Geometry check sheet. Reference: the model listing, model coordinates, mm. Face numbers are marked on the shaded views. A direction names the side the tool comes from. Round coordinates to 2 decimals unless told otherwise and drop trailing zeros. Order: outer loops, then holes, each group sorted by start corner. A loop starts at its lowest first (then second) coordinate and runs counter-clockwise, first axis right, second up. Notation, with made-up numbers: (46.25, -24) - (59.25, -24) arc R26 ccw to (59.25, 5) - close; hole circle Ø10 at (32, 58.5). An arc over 180 degrees is marked (long way). Return JSON: item names as keys, results as strings. Group by question number.
Q1. Sectioned sample at A-A, the plane y = 15.75. Record the cut outline in (x, z).
Q2. Material ranges on line 1 along Z through (x, y) = (7.5, 1.1); line 2 along X through (y, z) = (7.75, -28); line 3 along X through (y, z) = (21, -21), recorded low to high.
Q3. Tool access check on the marked faces 5 and 6. Record the directions out of +Z, -Z, +X, -X, +Y, -Y that give a thin tool (end or side, any length) a straight path to the whole face; none if there is none.
Q4. Sectioned sample at C-C, the plane x = 21.5. Record the cut outline in (y, z).
Q5. Gauge pin test, flat ends, axial feed: pin 1 Ø3 at (x, y) = (45, 14) entering from +Z (3 decimals); pin 2 Ø2.5 at (y, z) = (7.5, -5) entering from +X; pin 3 Ø8 at (x, z) = (43, -34) entering from +Y; pin 4 Ø3 at (x, z) = (64.5, -5.78) entering from +Y. Record the tip position at first contact, or that the pin passes through.
Q6. Sectioned sample at D-D, the plane z = -6. Record the cut outline in (x, y), then the cut area to 3 significant figures.
Q7. Sectioned sample at B-B, the plane z = -21. Record the cut outline in (x, y), then the cut area to 3 significant figures.
Q8. Draft check along X on the marked faces 1, 2, 3 and 4. Enter one of: pulls with the +X half, pulls with the -X half, needs draft (parallel to the pull), parting line crosses it, or undercut.
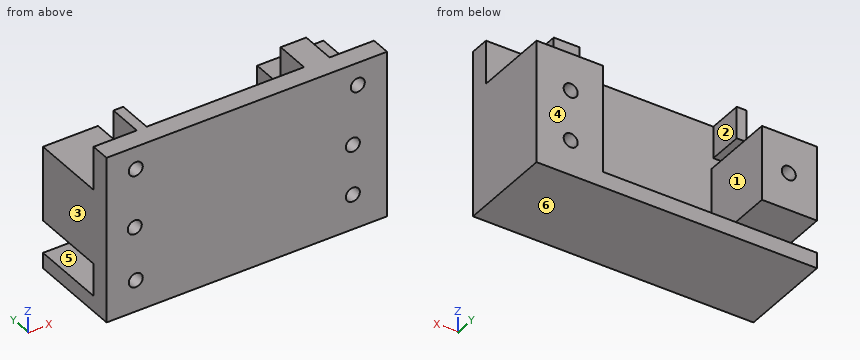
```python
from build123d import *

# Parameters (mm, degrees)
SKETCH2_W                = 72
SKETCH2_H                = 40
BOSS_EXTRUDE1_DEPTH      = 5
BOSS_EXTRUDE2_DEPTH      = 19.5
BOSS_EXTRUDE2_DEPTH_BACK = 5
SKETCH3_W                = 14.135898402
SKETCH3_H                = 19.186853455
CUT_EXTRUDE1_START       = 19.5
SKETCH4_R                = 1.8
CUT_EXTRUDE1_DEPTH       = 30
SKETCH8_W                = 2.527236714
SKETCH8_H                = 8.177193873
SKETCH8_W_2              = 6.563624393
BOSS_EXTRUDE7_DEPTH      = 9
SKETCH9_R                = 1.8
CUT_EXTRUDE2_DEPTH       = 53


with BuildPart() as part:
    # Sketch2 → Boss-Extrude1 (new body)
    with BuildSketch(Plane(origin=(0, 0, 0), x_dir=(1, 0, 0), z_dir=(0, 1, 0))):
        with Locations((36, 20)):
            Rectangle(SKETCH2_W, SKETCH2_H)
    extrude(amount=BOSS_EXTRUDE1_DEPTH)

    # Sketch3 → Boss-Extrude2 (add, two sides: drawn at the far end of the back side and taken through both)
    with BuildSketch(Plane(origin=(0, 5, 0), x_dir=(1, 0, 0), z_dir=(0, 1, 0)).offset(-BOSS_EXTRUDE2_DEPTH_BACK)):
        with Locations((7.067949201, 20.793426728)):
            Rectangle(SKETCH3_W, SKETCH3_H)
        Polygon((55, 38.754979203), (55, 11.2), (72, 11.2), (72, 42.754979203), (0, 42.754979203), (0, 38.754979203), align=None)
    extrude(amount=BOSS_EXTRUDE2_DEPTH + BOSS_EXTRUDE2_DEPTH_BACK)

    # Sketch4 → Cut-Extrude1 (cut)
    with BuildSketch(Plane(origin=(0, 5, 0), x_dir=(1, 0, 0), z_dir=(0, 1, 0)).offset(CUT_EXTRUDE1_START)):
        with Locations(Location((7.5, 34.648486257, 0), (0, 0, 90))):
            Circle(SKETCH4_R)
        with Locations(Location((7.5, 5.778304463, 0), (0, 0, 90))):
            Circle(SKETCH4_R)
        with Locations(Location((64.5, 5.778304463, 0), (0, 0, 90))):
            Circle(SKETCH4_R)
    extrude(amount=-CUT_EXTRUDE1_DEPTH, mode=Mode.SUBTRACT)

    # Sketch8 → Boss-Extrude7 (add)
    with BuildSketch(Plane(origin=(0, 5, 0), x_dir=(1, 0, 0), z_dir=(0, 1, 0))):
        with Locations((12.356862163, 4.088596937)):
            Rectangle(SKETCH8_W, SKETCH8_H)
        with Locations((57.312199978, 4.088596937)):
            Rectangle(SKETCH8_W_2, SKETCH8_H)
    extrude(amount=BOSS_EXTRUDE7_DEPTH)

    # Sketch9 → Cut-Extrude2 (cut)
    with BuildSketch(Plane(origin=(0, 24.5, 0), x_dir=(1, 0, 0), z_dir=(0, 1, 0))):
        with Locations(Location((7.244076977, 20.809705714, 0), (0, 0, 270))):
            Circle(SKETCH9_R)
        with Locations(Location((63.234445615, 20.809705714, 0), (0, 0, 270))):
            Circle(SKETCH9_R)
        with Locations(Location((63.234445615, 33.7549792, 0), (0, 0, 270))):
            Circle(SKETCH9_R)
    extrude(amount=-CUT_EXTRUDE2_DEPTH, mode=Mode.SUBTRACT)


solid = part.part
```
Reply:
{
 "1": {"outline": "(0, -42.75) - (72, -42.75) - (72, -11.2) - (55, -11.2) - (55, -38.75) - (0, -38.75) - close; (0, -30.39) - (14.14, -30.39) - (14.14, -11.2) - (0, -11.2) - close; hole circle Ø3.6 at (7.24, -20.81); hole circle Ø3.6 at (63.23, -33.75); hole circle Ø3.6 at (63.23, -20.81)"},
 "2": {"line 1": "-42.75 to -36.45, -32.85 to -22.59, -19.03 to -7.58, -3.98 to 0", "line 2": "0 to 14.14, 55 to 72", "line 3": "0 to 5.45, 9.03 to 14.14, 55 to 61.44, 65.02 to 72"},
 "3": {"face 5": "-X, +Y", "face 6": "-Z, +X, -X, +Y, -Y"},
 "4": {"outline": "(0, -42.75) - (24.5, -42.75) - (24.5, -38.75) - (5, -38.75) - (5, 0) - (0, 0) - close"},
 "5": {"pin 1": "z = -38.755", "pin 2": "x = 60.59", "pin 3": "y = 5", "pin 4": "through"},
 "6": {"outline": "(0, 0) - (5.71, 0) - (5.71, 5) - (0, 5) - close; (9.29, 0) - (62.71, 0) - (62.71, 5) - (60.59, 5) - (60.59, 14) - (54.03, 14) - (54.03, 5) - (13.62, 5) - (13.62, 14) - (11.09, 14) - (11.09, 5) - (9.29, 5) - close; (66.29, 0) - (72, 0) - (72, 5) - (66.29, 5) - close", "area": "406 mm^2"},
 "7": {"outline": "(0, 0) - (5.45, 0) - (5.45, 24.5) - (0, 24.5) - close; (9.03, 0) - (61.44, 0) - (61.44, 24.5) - (55, 24.5) - (55, 5) - (14.14, 5) - (14.14, 24.5) - (9.03, 24.5) - close; (65.02, 0) - (72, 0) - (72, 24.5) - (65.02, 24.5) - close", "area": "792 mm^2"},
 "8": {"face 1": "undercut", "face 2": "undercut", "face 3": "pulls with the -X half", "face 4": "needs draft"}
}
